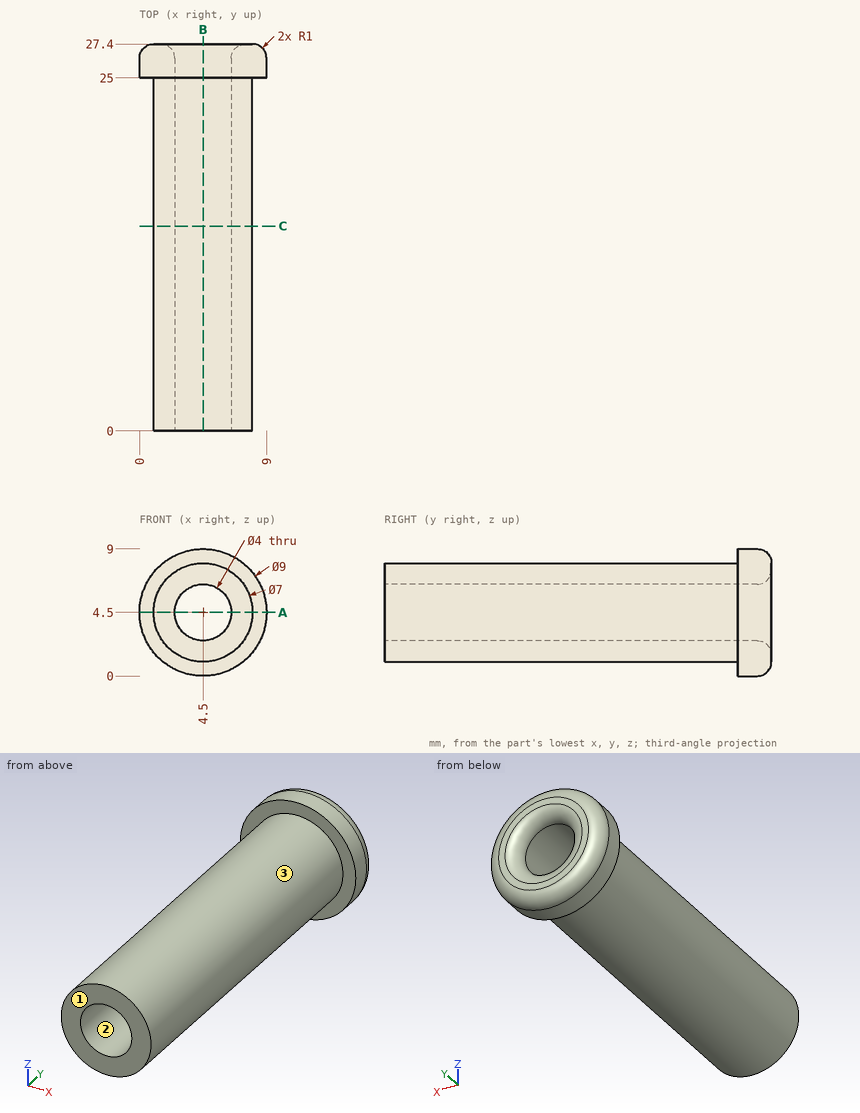
Drawing for the job (mm, zero at the part's lowest x, y, z). Coordinates: 2 decimals unless noted, no trailing zeros. Loops run counter-clockwise (first coordinate to the right, second up) from the corner with the lowest first, then second, coordinate; pieces in that order, holes last. Notation, with made-up numbers: (-34.5, 62.5) - (-24.5, 62.5) arc R16 ccw to (-24.5, 86.5) - close; hole circle Ø11 at (-39, -30.75). An arc over 180 degrees is marked (long way). Return JSON: item names as keys, results as strings.
1. Probe L1, parallel to Z at x = 4.5, y = 11; L2, parallel to Z at x = 2.75, y = 24.25. List the from-to ranges inside material, lowest first. Write a range as from..to.
Result:
{"L1": "z = 1..2.5, 6.5..8", "L2": "z = 1.47..3.53, 5.47..7.53"}
2. Drop flat-ended pins along their axis: pin 1 (4.5 mm diameter, centred on x = 4.5, z = 4.5, fed in from +Y); pin 2 (2 mm diameter, centred on y = 6.5, z = 4, fed in from +X); pin 3 (1.5 mm diameter, centred on y = 16.5, z = 5, fed in from -X). Give the stop position or say it passes through.
Result:
{"pin 1": "stops at y = 27.06", "pin 2": "stops at x = 8", "pin 3": "stops at x = 1"}
3. Band-saw the part on C-C (y = 14.5). Give the cut face in (x, z), and give its area (3 significant figures).
Result:
{"outline": "circle Ø7 at (4.5, 4.5); hole circle Ø4 at (4.5, 4.5)", "area": "25.9 mm2"}
4. Mould opens along X. For the marked faces 1, 2 and 3 say: released by +X, released by -X, zero draft, split by the parting line, or undercut.
Result:
{"face 1": "zero draft", "face 2": "undercut", "face 3": "split by the parting line"}
5. Band-saw the part on A-A (z = 4.5). Give the cut face in (x, y), and give its area (3 significant figures).
Result:
{"outline": "(0, 25) - (1, 25) - (1, 0) - (2.5, 0) - (2.5, 26.4) arc R1 ccw to (1.5, 27.4) - (1, 27.4) arc R1 ccw to (0, 26.4) - close; (6.5, 0) - (8, 0) - (8, 25) - (9, 25) - (9, 26.4) arc R1 ccw to (8, 27.4) - (7.5, 27.4) arc R1 ccw to (6.5, 26.4) - close", "area": "86.1 mm2"}
6. Band-saw the part on B-B (x = 4.5). Give the cut face in (y, z).
Result:
{"outline": "(0, 1) - (25, 1) - (25, 0) - (26.4, 0) arc R1 ccw to (27.4, 1) - (27.4, 1.5) arc R1 ccw to (26.4, 2.5) - (0, 2.5) - close; (0, 6.5) - (26.4, 6.5) arc R1 ccw to (27.4, 7.5) - (27.4, 8) arc R1 ccw to (26.4, 9) - (25, 9) - (25, 8) - (0, 8) - close"}
